```python
from build123d import *

# Parameters (mm, degrees)
SKETCH1_W           = 914.4
SKETCH1_H           = 609.6
SKETCH1_W_2         = 863.6
SKETCH1_H_2         = 558.8
BOSS_EXTRUDE1_DEPTH = 12.7
SKETCH2_W           = 25.4
SKETCH2_H           = 25.4
BOSS_EXTRUDE2_DEPTH = 381
SKETCH3_W           = 914.4
SKETCH3_H           = 609.6
SKETCH3_W_2         = 863.6
SKETCH3_H_2         = 558.8
BOSS_EXTRUDE3_DEPTH = 25.4


with BuildPart() as part:
    # Sketch1 → Boss-Extrude1 (new body, symmetric)
    with BuildSketch(Plane(origin=(0, 0, 0), x_dir=(0, 0, -1), z_dir=(0, 1, 0))):
        with Locations((457.2, 304.8)):
            Rectangle(SKETCH1_W, SKETCH1_H)
        with Locations((457.2, 304.8)):
            Rectangle(SKETCH1_W_2, SKETCH1_H_2, mode=Mode.SUBTRACT)
    extrude(amount=BOSS_EXTRUDE1_DEPTH, both=True)

    # Sketch2 → Boss-Extrude2 (add)
    with BuildSketch(Plane(origin=(0, 12.7, 0), x_dir=(0, 0, -1), z_dir=(0, 1, 0))):
        with Locations((12.7, 596.9)):
            Rectangle(SKETCH2_W, SKETCH2_H)
        with Locations((901.7, 596.9)):
            Rectangle(SKETCH2_W, SKETCH2_H)
        with Locations((901.7, 12.7)):
            Rectangle(SKETCH2_W, SKETCH2_H)
        with Locations((12.7, 12.7)):
            Rectangle(SKETCH2_W, SKETCH2_H)
    extrude(amount=BOSS_EXTRUDE2_DEPTH)

    # Sketch3 → Boss-Extrude3 (add)
    with BuildSketch(Plane(origin=(0, 393.7, 0), x_dir=(0, 0, -1), z_dir=(0, 1, 0))):
        with Locations((457.2, 304.8)):
            Rectangle(SKETCH3_W, SKETCH3_H)
        with Locations((457.2, 304.8)):
            Rectangle(SKETCH3_W_2, SKETCH3_H_2, mode=Mode.SUBTRACT)
    extrude(amount=-BOSS_EXTRUDE3_DEPTH)


solid = part.part
```
The listing builds one solid part. Answer for the finished solid, in the listing's coordinates (mm). A direction names the side the tool comes from. Coordinates: 2 decimals unless noted, no trailing zeros. Write each loop counter-clockwise with the first axis right and the second up, starting at its lowest first coordinate (ties: lowest second). Pieces come first, ordered by that corner, then holes. Notation, with made-up numbers: (14, 9) - (48, 9) arc R30 cw to (48, 45) - close; hole circle Ø3 at (60, 35). An arc over 180 degrees is marked (long way). Return JSON: item names as keys, results as strings. Group by question number.
1. A cutting plane is placed at A-A, the plane x = -513.5. Determine the outline of the cut face in (y, z).
2. Which of the six approach directions +Z, -Z, +X, -X, +Y, -Y give full straight-line access (tool end or side, diameter ignored) to faces 1 (the flat face through (-25.4, 188, -13)), 2 (the flat face through (-13, 393.7, -421)), 3 (the flat face through (-301, 381, -25.4)), 4 (the flat face through (-13, 368.3, -451))?
3. A cutting plane is placed at B-B, the plane z = -245. Determine the outline of the cut face in (x, y), plus the area to 3 significant figures.
4. Determine the mould class of faces 5 (the flat face through (-281, 11, -914.4)), 6 (the flat face through (-281, 370, 0)), 7 (the flat face through (-301, 0, -889)), 8 (the flat face through (-309, 12.7, -902)) for opening direction Z: released by +Z, released by -Z, zero draft, split by the parting line, or undercut.
5. Straight lines are drawn through the part: L1, parallel to Z at x = -59.5, y = 370.5; L2, parallel to X at y = 8, z = -81.5; L3, parallel to Y at x = -25, z = -286.5. For each, find the intervals that lie inside material, in ascending order.
Ans:
{
 "1": {"outline": "(-12.7, -914.4) - (12.7, -914.4) - (12.7, -889) - (-12.7, -889) - close; (-12.7, -25.4) - (12.7, -25.4) - (12.7, 0) - (-12.7, 0) - close; (368.3, -914.4) - (393.7, -914.4) - (393.7, -889) - (368.3, -889) - close; (368.3, -25.4) - (393.7, -25.4) - (393.7, 0) - (368.3, 0) - close"},
 "2": {"face 1": "+Z, -Z", "face 2": "+Z, -Z, +X, -X, +Y", "face 3": "+Y, -Y", "face 4": "+X, -X"},
 "3": {"outline": "(-609.6, -12.7) - (-584.2, -12.7) - (-584.2, 12.7) - (-609.6, 12.7) - close; (-609.6, 368.3) - (-584.2, 368.3) - (-584.2, 393.7) - (-609.6, 393.7) - close; (-25.4, -12.7) - (0, -12.7) - (0, 12.7) - (-25.4, 12.7) - close; (-25.4, 368.3) - (0, 368.3) - (0, 393.7) - (-25.4, 393.7) - close", "area": "2,580 mm²"},
 "4": {"face 5": "released by -Z", "face 6": "released by +Z", "face 7": "undercut", "face 8": "zero draft"},
 "5": {"L1": "-914.4 to -889, -25.4 to 0", "L2": "-609.6 to -584.2, -25.4 to 0", "L3": "-12.7 to 12.7, 368.3 to 393.7"}
}
